Design review of the part built by this model. Coordinates are the model's own, in mm. A direction names the side the tool comes from. Round coordinates to 2 decimals unless told otherwise and drop trailing zeros. Order: outer loops, then holes, each group sorted by start corner. A loop starts at its lowest first (then second) coordinate and runs counter-clockwise, first axis right, second up. Notation, with made-up numbers: (-35.5, 42) - (21.5, 42) arc R20 cw to (21.5, 75) - close; hole circle Ø9 at (-0.75, 66.5). An arc over 180 degrees is marked (long way). Use CSV: the item, a comma, the result in double quotes.
from build123d import *

# Parameters (mm, degrees)
SKETCH1_R           = 75
BOSS_EXTRUDE1_DEPTH = 2.9
SKETCH2_R           = 1.6
SKETCH2_R_2         = 1.4
SKETCH2_W           = 60
SKETCH2_H           = 6
CUT_EXTRUDE1_DEPTH  = 10
CUT_EXTRUDE2_DEPTH  = 3.9


with BuildPart() as part:
    # Sketch1 → Boss-Extrude1 (new body)
    with BuildSketch(Plane(origin=(0, 0, 0), x_dir=(1, 0, 0), z_dir=(0, 1, 0))):
        Circle(SKETCH1_R)
    extrude(amount=BOSS_EXTRUDE1_DEPTH)

    # Sketch2 → Cut-Extrude1 (cut)
    with BuildSketch(Plane(origin=(0, 2.9, 0), x_dir=(1, 0, 0), z_dir=(0, 1, 0))):
        with BuildLine():
            ThreePointArc((-68.72850121, -30.023209712), (-54.08520342, 0), (-68.72850121, 30.023209712))
            ThreePointArc((-68.72850121, 30.023209712), (-75, 0), (-68.72850121, -30.023209712))
        make_face()
        with BuildLine():
            ThreePointArc((75, 0), (73.415385277, 15.335618821), (68.72850121, 30.023209712))
            ThreePointArc((68.72850121, 30.023209712), (54.08520342, 0), (68.72850121, -30.023209712))
            ThreePointArc((68.72850121, -30.023209712), (73.415385277, -15.335618821), (75, 0))
        make_face()
        with Locations((9.1, -24.090757895)):
            Circle(SKETCH2_R)
        with Locations((40.3, -24.090757895)):
            Circle(SKETCH2_R)
        with Locations((40.3, -4.890757895)):
            Circle(SKETCH2_R)
        with Locations((40.3, 14.309242105)):
            Circle(SKETCH2_R)
        with Locations((9.1, 14.309242105)):
            Circle(SKETCH2_R)
        with Locations((9.1, -4.890757895)):
            Circle(SKETCH2_R)
        with Locations((-9.1, 4.890757895)):
            Circle(SKETCH2_R)
        with Locations((-9.1, -14.309242105)):
            Circle(SKETCH2_R)
        with Locations((-9.1, 24.090757895)):
            Circle(SKETCH2_R)
        with Locations((-40.3, 24.090757895)):
            Circle(SKETCH2_R)
        with Locations((-40.3, 4.890757895)):
            Circle(SKETCH2_R)
        with Locations((-40.3, -14.309242105)):
            Circle(SKETCH2_R)
        with Locations((-22.14, -46.709242105)):
            Circle(SKETCH2_R_2)
        with Locations((-2.56, -46.709242105)):
            Circle(SKETCH2_R_2)
        with Locations((22.14, 46.709242105)):
            Circle(SKETCH2_R_2)
        with Locations((2.56, 46.709242105)):
            Circle(SKETCH2_R_2)
        with Locations((0, -58.709242105)):
            Rectangle(SKETCH2_W, SKETCH2_H)
        with Locations((0, 58.709242105)):
            Rectangle(SKETCH2_W, SKETCH2_H)
    extrude(amount=-CUT_EXTRUDE1_DEPTH, mode=Mode.SUBTRACT)

    # Sketch3 → Cut-Extrude2 (cut, through all)
    with BuildSketch(Plane(origin=(0, 2.9, 0), x_dir=(1, 0, 0), z_dir=(0, 1, 0))):
        with BuildLine():
            Line((-51.177473943, 2.65), (-54.177473943, 2.65))
            ThreePointArc((-54.177473943, 2.65), (-54.08520342, 0), (-54.177473943, -2.65))
            Line((-54.177473943, -2.65), (-51.177473943, -2.65))
            Line((-51.177473943, -2.65), (-51.177473943, 2.65))
        make_face()
    extrude(amount=-CUT_EXTRUDE2_DEPTH, mode=Mode.SUBTRACT)


solid = part.part
1) We need section B-B (z = -59). Give the boundary of the cut face in (x, y).
Data:
outline,"(-46.3, 0) - (-30, 0) - (-30, 2.9) - (-46.3, 2.9) - close; (30, 0) - (46.3, 0) - (46.3, 2.9) - (30, 2.9) - close"
2) We need section D-D (z = 40). Give the boundary of the cut face in (x, y), then the cut area to 3 significant figures.
Data:
outline,"(-63.44, 0) - (63.44, 0) - (63.44, 2.9) - (-63.44, 2.9) - close"
area,"368 mm2"
3) To check wall thickness, follow L1, parallel to Z at x = -40.3, y = 1.85; L2, parallel to Z at x = -10, y = 2.5; L3, parallel to Z at x = -20, y = 1.4. State the ranges of each line that lie inside material, in increasing order. Write a range as from..to.
Data:
L1,"z = -63.25..-25.69, -22.49..-6.49, -3.29..12.71, 15.91..63.25"
L2,"z = -74.33..-61.71, -55.71..-25.41, -22.77..-6.21, -3.57..12.99, 15.63..55.71, 61.71..74.33"
L3,"z = -72.28..-61.71, -55.71..55.71, 61.71..72.28"
4) We need section A-A (y = 0.65). Give the number of separate pieces and of enclosed holes in the cut face, then the cut area to 3 significant figures.
Data:
separate pieces,"1"
enclosed holes,"18"
area,"15,100 mm2"
5) Insertion check: pin 1 Ø4.5 at (x, z) = (-2.56, 46.71) entering from +Y; pin 2 Ø0.9 at (y, z) = (1, -58.5) entering from +X; pin 3 Ø1.4 at (x, y) = (-7, 2) entering from +Z; pin 4 Ø1.4 at (x, y) = (13, 1) entering from -Z. Each pin has a flat end and moves straight along its axis. Give the tip position at first contact, or say it passes through.
Data:
pin 1,"stops at y = 2.9"
pin 2,"stops at x = 47.49"
pin 3,"stops at z = 74.73"
pin 4,"stops at z = -73.98"
6) We need section C-C (z = 11). Give the boundary of the cut face in (x, y).
Data:
outline,"(-55.71, 0) - (55.71, 0) - (55.71, 2.9) - (-55.71, 2.9) - close"
7) For faces 5 (the face through (-58.65, 1.47, 18.08)), 6 (the face through (-41.9, 1.47, -4.96)), list the 3-axis set-ups (+Z, -Z, +X, -X, +Y, -Y) from which the entire face can be reached by the end or side of a thin tool; tool diameter is ignored.
Data:
face 5,"-X, +Y, -Y"
face 6,"+Y, -Y"
8) The part is to be moulded in two halves that separate along X. For faces 1 (the face through (-58.44, 1.47, -17.69)), 2 (the face through (-9.308, 1.47, -6.477)), 3 (the face through (54.09, 1.47, -0.48)), 4 (the face through (-1, 2.9, -1)), say which applies: +X half, -X half, draft (parallel to the pull), parting line (faces both ways), or undercut.
Data:
face 1,"-X half"
face 2,"undercut"
face 3,"+X half"
face 4,"draft"
